from build123d import *

# Parameters (mm, degrees)
F1_DEPTH = 25.4


with BuildPart() as f1:
    # F0 (on Front) → F1 (new body)
    with BuildSketch(Plane.XZ):
        with BuildLine():
            Line((-12.4426856389, -12.9730125086), (-13.1896968379, -5.4903274543))
            ThreePointArc((-13.1896968379, -5.4903274543), (-0.1668346208, -12.2836148574), (7.8865187243, 0))
            Line((7.8865187243, 0), (10.5906810166, -13.0574683954))
            Line((10.5906810166, -13.0574683954), (14.8144917242, -13.957073912))
            Line((14.8144917242, -13.957073912), (18.4332933277, 3.033854533))
            Line((18.4332933277, 3.033854533), (7.791120559, 5.3004706278))
            Line((7.791120559, 5.3004706278), (7.791120559, 21.074494347))
            Line((7.791120559, 21.074494347), (12.3297581449, 18.2102192193))
            Line((12.3297581449, 18.2102192193), (18.2683356106, 18.2102192193))
            Line((18.2683356106, 18.2102192193), (12.3297581449, 28.7676900625))
            Line((12.3297581449, 28.7676900625), (7.380944211, 28.4377671778))
            Line((7.380944211, 28.4377671778), (7.380944211, 41.1397255957))
            Line((7.380944211, 41.1397255957), (21.8974649906, 41.3046851754))
            Line((21.8974649906, 41.3046851754), (17.9384145886, 51.6971945763))
            Line((17.9384145886, 51.6971945763), (7.380944211, 51.6971945763))
            ThreePointArc((7.380944211, 51.6971945763), (5.8269963178, 52.5462179029), (4.209248367, 53.2662777833))
            ThreePointArc((4.209248367, 53.2662777833), (2.1348058911, 53.9718233781), (0, 54.4654932873))
            ThreePointArc((0, 54.4654932873), (-3.971449067, 54.80540535), (-7.938379177, 54.4162865973))
            ThreePointArc((-7.938379177, 54.4162865973), (-10.0209611702, 53.9098413782), (-12.0437239792, 53.2012758293))
            ThreePointArc((-12.0437239792, 53.2012758293), (-13.577773448, 52.5074144495), (-15.053678304, 51.6971945763))
            Line((-15.053678304, 51.6971945763), (-20.6623356789, 51.6971945763))
            Line((-20.6623356789, 51.6971945763), (-30.5599626154, 39.3251590431))
            Line((-30.5599626154, 39.3251590431), (-24.621386081, 39.3251590431))
            Line((-24.621386081, 39.3251590431), (-15.1529135182, 41.3046851754))
            Line((-15.1529135182, 41.3046851754), (-15.1529135182, 28.7676900625))
            Line((-15.1529135182, 28.7676900625), (-19.177692011, 28.7676900625))
            Line((-19.177692011, 28.7676900625), (-24.621386081, 16.560614109))
            Line((-24.621386081, 16.560614109), (-20.9508969498, 14.9237749517))
            Line((-20.9508969498, 14.9237749517), (-15.1529135182, 20.6647776067))
            Line((-15.1529135182, 20.6647776067), (-15.1529135182, 7.9636173323))
            Line((-15.1529135182, 7.9636173323), (-21.3221795857, 3.033854533))
            Line((-21.3221795857, 3.033854533), (-15.1529135182, -13.957073912))
            Line((-15.1529135182, -13.957073912), (-12.4426856389, -12.9730125086))
        make_face()
        with BuildLine():
            ThreePointArc((-13.1896968379, -5.4903274543), (-13.8154393629, -2.7802733754), (-13.7378070503, 0))
            Line((-13.7378070503, 0), (-13.1896968379, -5.4903274543))
        make_face(mode=Mode.SUBTRACT)
        with BuildLine():
            ThreePointArc((0, 54.4654932873), (2.1348058911, 53.9718233781), (4.209248367, 53.2662777833))
            Line((4.209248367, 53.2662777833), (7.8750308603, 61.7822111755))
            Line((7.8750308603, 61.7822111755), (0, 61.7822111755))
            Line((0, 61.7822111755), (0, 54.4654932873))
        make_face()
        with BuildLine():
            Line((-16.4149385959, 60.7384818016), (-12.0437239792, 53.2012758293))
            ThreePointArc((-12.0437239792, 53.2012758293), (-10.0209611702, 53.9098413782), (-7.938379177, 54.4162865973))
            Line((-7.938379177, 54.4162865973), (-12.8155713901, 62.8259405494))
            Line((-12.8155713901, 62.8259405494), (-16.4149385959, 60.7384818016))
        make_face()
        with BuildLine():
            Line((-13.1896968379, -5.4903274543), (-13.7378070503, 0))
            ThreePointArc((-13.7378070503, 0), (-13.8154393629, -2.7802733754), (-13.1896968379, -5.4903274543))
        make_face()
    extrude(amount=F1_DEPTH)


solid = f1.part
Design review of the part built by this model. Coordinates are the model's own, in mm. A direction names the side the tool comes from. Coordinates: 2 decimals unless noted, no trailing zeros. Order: outer loops, then holes, each group sorted by start corner. A loop starts at its lowest first (then second) coordinate and runs counter-clockwise, first axis right, second up.
Item 1: The part is to be moulded in two halves that separate along X. For faces 1 (the flat face through (-28, -13, 39.325)), 2 (the flat face through (16.6, -12.52, -5.58)), 3 (the flat face through (-13.817, -12.522, -13.472)), say which applies: pulls with the +X half, pulls with the -X half, needs draft (parallel to the pull), parting line crosses it, or undercut.
Item 2: For line 1 (X direction, y = -12.5, z = 19.5); line 2 (X direction, y = -11.5, z = 34); line 3 (Z direction, x = 13, y = -14.25), list the stretches that pass through material, from the lowest coordinate up.
Item 3: For pin 1 Ø2.5 at (x, y) = (4.5, -17) entering from +Z; pin 2 Ø5 at (x, y) = (-12, -5) entering from -Z; pin 3 Ø1.5 at (x, z) = (-16.5, 10) entering from +Y; pin 4 Ø6 at (x, y) = (-18, -15.5) entering from +Z, all flat-tipped, find the tip position at first contact; note any pin that passes through.
Item 4: For faces 4 (the flat face through (-10.34, -12.52, 58.56)), 5 (the flat face through (15.34, -12.52, 23.42)), 6 (the flat face through (-19.95, -12.52, 40.3)), 7 (the flat face through (-18.194, -12.522, 5.533)), 8 (the flat face through (19.946, -12.522, 46.428)), list the 3-axis set-ups (+Z, -Z, +X, -X, +Y, -Y) from which the entire face can be reached by the end or side of a thin tool; tool diameter is ignored.
Item 5: Take a section at C-C, the plane z = 36. Write out the cut boundary in (x, y), then the cut area to 3 significant figures.
Item 6: Take a section at A-A, the plane x = -14. Write out the cut boundary in (y, z).
Item 7: Take a section at B-B, the plane z = 9.5. Write out the cut boundary in (x, y), then the cut area to 3 significant figures.
The answers:
1. face 1: needs draft
1. face 2: pulls with the +X half
1. face 3: undercut
2. line 1: x = -23.31 to -16.33, -15.15 to 7.79, 10.29 to 17.54
2. line 2: x = -15.15 to 7.38
2. line 3: z = -13.57 to 4.19, 18.21 to 27.58, 41.2 to 51.7
3. pin 1: stops at z = 61.78
3. pin 2: stops at z = -13.72
3. pin 3: passes through
3. pin 4: stops at z = 61.56
4. face 4: +Z, +Y, -Y
4. face 5: +X, +Y, -Y
4. face 6: +Y, -Y
4. face 7: -X, +Y, -Y
4. face 8: +Z, +X, +Y, -Y
5. outline: (-15.15, -25.4) - (7.38, -25.4) - (7.38, 0) - (-15.15, 0) - close
5. area: 572 mm2
6. outline: (-25.4, -13.54) - (0, -13.54) - (0, 52.29) - (-25.4, 52.29) - close; (-25.4, 56.57) - (0, 56.57) - (0, 62.14) - (-25.4, 62.14) - close
7. outline: (-15.15, -25.4) - (7.79, -25.4) - (7.79, 0) - (-15.15, 0) - close
7. area: 583 mm2
